Design review of the part shown in the three views and the two pictorial views. Dimensions are in mm from the part's minimum x, y and z. A direction names the side the tool comes from. Give positions to 0.01 mm unless a question says otherwise; leave off trailing zeros. Loops run counter-clockwise (first coordinate to the right, second up) from the corner with the lowest first, then second, coordinate; pieces in that order, holes last.
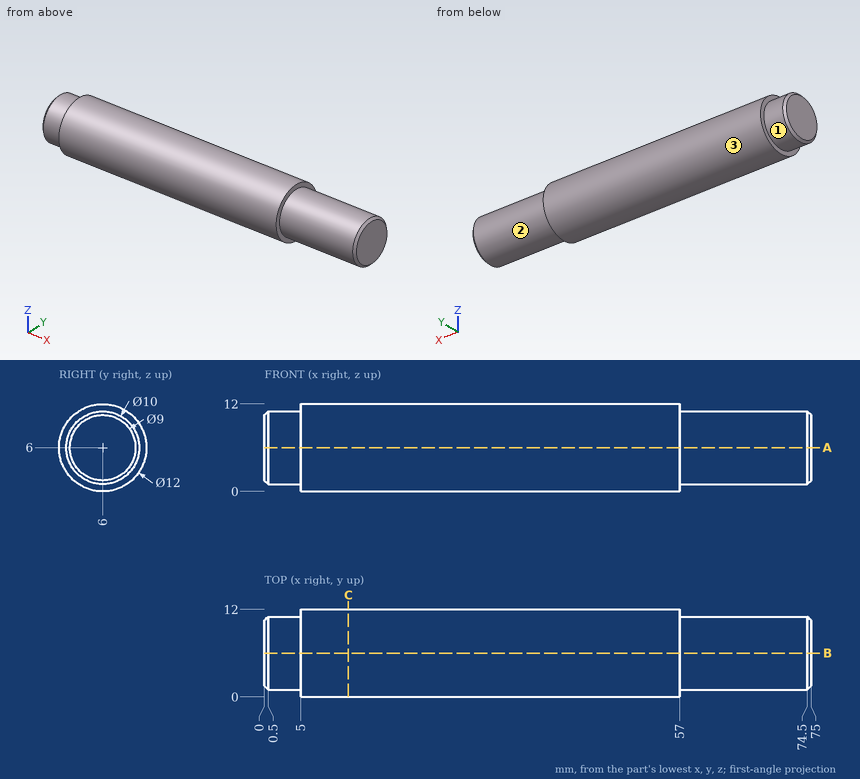
Q1. Machinability: for the marked faces 1, 2 and 3, which of the approach directions +Z, -Z, +X, -X, +Y, -Y give a long, thin tool a straight path to every point of the face, cutting with its end or side? Answer none if there is none.
Answers:
face 1: -X
face 2: +X
face 3: +X, -X
Q2. Consider section A-A on z = 6. Give the boundary of the cut face in (x, y).
Answers:
outline: (0, 1.5) - (0.5, 1) - (5, 1) - (5, 0) - (57, 0) - (57, 1) - (74.5, 1) - (75, 1.5) - (75, 10.5) - (74.5, 11) - (57, 11) - (57, 12) - (5, 12) - (5, 11) - (0.5, 11) - (0, 10.5) - close
Q3. For probe 1 along X at (y, z) = (10.75, 8.75); probe 2 along Y at (x, z) = (44, 11.25); probe 3 along Z at (x, y) = (27, 5.25), list the stretches that pass through material, from the lowest coordinate up.
Answers:
probe 1: x = 5 to 57
probe 2: y = 3.1 to 8.9
probe 3: z = 0.05 to 11.95
Q4. For pin 1 Ø1 at (x, y) = (67, 9.5) entering from -Z; pin 2 Ø3 at (x, z) = (36, 2) entering from +Y; pin 3 Ø1 at (x, y) = (44.5, 7.5) entering from +Z; pin 4 Ø3.5 at (y, z) = (4, 6) entering from -X, all flat-tipped, find the tip position at first contact; note any pin that passes through.
Answers:
pin 1: stops at z = 2
pin 2: stops at y = 11.45
pin 3: stops at z = 11.92
pin 4: stops at x = 0
Q5. Consider section C-C on x = 11.5. Give the boundary of the cut face in (y, z).
Answers:
outline: circle Ø12 at (6, 6)
